```python
from build123d import *

# Parameters (mm, degrees)
BOSS_EXTRUDE1_DEPTH = 50
SKETCH2_R           = 10
CUT_EXTRUDE1_DEPTH  = 51
SKETCH3_W           = 90
SKETCH3_H           = 5
CUT_EXTRUDE2_DEPTH  = 51


with BuildPart() as part:
    # Sketch1 → Boss-Extrude1 (new body)
    with BuildSketch(Plane(origin=(0, 0, 0), x_dir=(0, 0, -1), z_dir=(1, 0, 0))):
        Polygon((40, 70), (0, 40), (0, 0), (100, 0), (100, 70), align=None)
    extrude(amount=BOSS_EXTRUDE1_DEPTH)

    # Sketch2 → Cut-Extrude1 (cut, through all)
    with BuildSketch(Plane(origin=(50, 0, 0), x_dir=(0, 0, -1), z_dir=(1, 0, 0))):
        with Locations((50, 35)):
            Circle(SKETCH2_R)
    extrude(amount=-CUT_EXTRUDE1_DEPTH, mode=Mode.SUBTRACT)

    # Sketch3 → Cut-Extrude2 (cut, through all)
    with BuildSketch(Plane(origin=(50, 0, 0), x_dir=(0, 0, -1), z_dir=(1, 0, 0))):
        with Locations((50, 7.5)):
            Rectangle(SKETCH3_W, SKETCH3_H)
    extrude(amount=-CUT_EXTRUDE2_DEPTH, mode=Mode.SUBTRACT)


solid = part.part
```
Check sheet for the modelled part. Datum: model origin and axes. Units: mm. A direction names the side the tool comes from. Give positions to 0.01 mm unless a question says otherwise; leave off trailing zeros. Write each loop counter-clockwise with the first axis right and the second up, starting at its lowest first coordinate (ties: lowest second). Pieces come first, ordered by that corner, then holes. Notation, with made-up numbers: (65.25, 34.5) -> (85.25, 34.5) arc R23 ccw to (85.25, 71.5) -> close; hole circle Ø6 at (57, -24.5). An arc over 180 degrees is marked (long way). Use CSV: the item, a comma, the result in double quotes. Start each with the question number.
Q1. Tool access check on faces 5 (the flat face through (25, 0, -49)), 6 (the flat face through (25, 10, -49)). Record the directions out of +Z, -Z, +X, -X, +Y, -Y that give a thin tool (end or side, any length) a straight path to the whole face; none if there is none.
Q2. Release check for a two-part mould opening along Y. For faces 1 (the flat face through (25, 5, -49)), 2 (the flat face through (25, 70, -70)), 3 (the flat face through (50, 35.5, -60.4)), 4 (the cylindrical face through (25, 29, -42)) record: +Y half, -Y half, draft (parallel to the pull), parting line (faces both ways), or undercut.
Q3. Cross-section at C-C on y = 43. Enter the section's corners in (x, z).
Q4. Cross-section at D-D on x = 39. Enter the section's corners in (y, z), and give its area (3 significant figures).
Q5. Scan lines: line 1 along Y through (x, z) = (20, -50); line 2 along Z through (x, y) = (39, 7); line 3 along Y through (x, z) = (21, -89.5). Record each from-to range of solid material in increasing order.
Q6. Cross-section at B-B on z = -50. Enter the section's corners in (x, y), and give its area (3 significant figures).
Q7. Cross-section at A-A on z = -91. Enter the section's corners in (x, y).
Q8. Depth check by flat-ended pin: P1, Ø4, axis at x = 33.5, y = 50, coming from the +Z side. Enter the tip coordinate at first touch or a pass-through.
Working result:
1,face 5,"+Z, -Z, +X, -X, -Y"
1,face 6,"+X, -X"
2,face 1,"undercut"
2,face 2,"+Y half"
2,face 3,"draft"
2,face 4,"undercut"
3,outline,"(0, -100) -> (50, -100) -> (50, -56) -> (0, -56) -> close; (0, -44) -> (50, -44) -> (50, -4) -> (0, -4) -> close"
4,outline,"(0, -100) -> (70, -100) -> (70, -40) -> (40, 0) -> (0, 0) -> close; hole (5, -95) -> (10, -95) -> (10, -5) -> (5, -5) -> close; hole circle Ø20 at (35, -50)"
4,area,"5,640 mm^2"
5,line 1,"y = 0 to 5, 10 to 25, 45 to 70"
5,line 2,"z = -100 to -95, -5 to 0"
5,line 3,"y = 0 to 5, 10 to 70"
6,outline,"(0, 0) -> (50, 0) -> (50, 5) -> (0, 5) -> close; (0, 10) -> (50, 10) -> (50, 25) -> (0, 25) -> close; (0, 45) -> (50, 45) -> (50, 70) -> (0, 70) -> close"
6,area,"2,250 mm^2"
7,outline,"(0, 0) -> (50, 0) -> (50, 5) -> (0, 5) -> close; (0, 10) -> (50, 10) -> (50, 70) -> (0, 70) -> close"
8,P1,"stops at z = -10.67"
